Check sheet for the modelled part. Datum: model origin and axes. Units: mm. A direction names the side the tool comes from. Round coordinates to 2 decimals unless told otherwise and drop trailing zeros. Write each loop counter-clockwise with the first axis right and the second up, starting at its lowest first coordinate (ties: lowest second). Pieces come first, ordered by that corner, then holes. Notation, with made-up numbers: M -6.5,-17 L 10.5,-17 A12 cw 10.5,-9 Z; hole C 33.5,-19.5 d4. An arc over 180 degrees is marked long. Answer in a Markdown table with one row per item.
```python
from build123d import *

# Parameters (mm, degrees)
SKETCH1_W                = 34
SKETCH1_H                = 15
BOSS_EXTRUDE1_DEPTH      = 30
BOSS_EXTRUDE2_DEPTH      = 7
BOSS_EXTRUDE2_DEPTH_BACK = 37
CUT_EXTRUDE2_DEPTH       = 38
CUT_EXTRUDE3_DEPTH       = 6
CUT_EXTRUDE3_DEPTH_BACK  = 40
SKETCH7_R                = 2.75
CUT_EXTRUDE4_DEPTH       = 25.660254038


with BuildPart() as part:
    # Sketch1 → Boss-Extrude1 (new body)
    with BuildSketch(Plane.XY):
        with Locations((17, 7.5)):
            Rectangle(SKETCH1_W, SKETCH1_H)
    extrude(amount=BOSS_EXTRUDE1_DEPTH)

    # Sketch3 → Boss-Extrude2 (add, two sides)
    with BuildSketch(Plane.XY.offset(30)) as boss_extrude2_sk:
        Polygon((0, 0), (-5, -8.660254038), (-5, -9.660254038), (39, -9.660254038), (39, -8.660254038), (34, 0), align=None)
    extrude(amount=BOSS_EXTRUDE2_DEPTH)
    extrude(boss_extrude2_sk.sketch, amount=-BOSS_EXTRUDE2_DEPTH_BACK)

    # Sketch5 → Cut-Extrude2 (cut, through all)
    with BuildSketch(Plane.XY.offset(30)):
        Polygon((8, 4.324573519), (10.75, 5.91228676), (10.75, 9.08771324), (8, 10.675426481), (5.25, 9.08771324), (5.25, 5.91228676), align=None)
        Polygon((26, 4.324573519), (28.75, 5.91228676), (28.75, 9.08771324), (26, 10.675426481), (23.25, 9.08771324), (23.25, 5.91228676), align=None)
    extrude(amount=-CUT_EXTRUDE2_DEPTH, mode=Mode.SUBTRACT)

    # Sketch6 → Cut-Extrude3 (cut, two sides)
    with BuildSketch(Plane.ZY) as cut_extrude3_sk:
        Polygon((30, 0), (37, -8.660254038), (37, 0), align=None)
        Polygon((0, 0), (-7, -8.660254038), (-7, 0), align=None)
    extrude(amount=CUT_EXTRUDE3_DEPTH, mode=Mode.SUBTRACT)
    extrude(cut_extrude3_sk.sketch, amount=-CUT_EXTRUDE3_DEPTH_BACK, mode=Mode.SUBTRACT)

    # Sketch7 → Cut-Extrude4 (cut, through all)
    with BuildSketch(Plane(origin=(0, 15, 0), x_dir=(1, 0, 0), z_dir=(0, 1, 0))):
        with Locations((17, -6)):
            Circle(SKETCH7_R)
        with Locations((17, -24)):
            Circle(SKETCH7_R)
    extrude(amount=-CUT_EXTRUDE4_DEPTH, mode=Mode.SUBTRACT)


solid = part.part
```
1. Section check C-C, the plane z = 2. Record the cut outline in (x, y).
Found:
| item | result |
|---|---|
| outline | M -5,-9.66 L 39,-9.66 L 39,-8.66 L 34,0 L 34,15 L 0,15 L 0,0 L -5,-8.66 Z; hole M 5.25,5.91 L 8,4.32 L 10.75,5.91 L 10.75,9.09 L 8,10.68 L 5.25,9.09 Z; hole M 23.25,5.91 L 26,4.32 L 28.75,5.91 L 28.75,9.09 L 26,10.68 L 23.25,9.09 Z |
2. Section check B-B, the plane x = 17. Record the cut outline in (y, z), and give its area (3 significant figures).
Found:
| item | result |
|---|---|
| outline | M -9.66,-7 L -8.66,-7 L 0,0 L 15,0 L 15,3.25 L -9.66,3.25 Z; M -9.66,8.75 L 15,8.75 L 15,21.25 L -9.66,21.25 Z; M -9.66,26.75 L 15,26.75 L 15,30 L 0,30 L -8.66,37 L -9.66,37 Z |
| area | 543 mm2 |
3. Go/stop test with flat-tipped pins: pin 1 (1.6 mm diameter, centred on y = 8, z = 12, fed in from -X); pin 2 (1.5 mm diameter, centred on x = 16.5, y = -0.5, fed in from +Z); pin 3 (10 mm diameter, centred on x = 0, y = -7, fed in from -Z); pin 4 (10 mm diameter, centred on y = -2.5, z = 13.5, fed in from +X). Record where each tip stops, or that it passes through.
Found:
| item | result |
|---|---|
| pin 1 | stops at x = 0 |
| pin 2 | stops at z = 31.01 |
| pin 3 | stops at z = -7 |
| pin 4 | stops at x = 38.33 |
4. Scan lines: L1, parallel to Z at x = 17, y = 9.5; L2, parallel to X at y = 8.25, z = 24; L3, parallel to Z at x = 16, y = -2.75. Record each from-to range of solid material in increasing order.
Found:
| item | result |
|---|---|
| L1 | z = 0 to 3.25, 8.75 to 21.25, 26.75 to 30 |
| L2 | x = 0 to 5.25, 10.75 to 14.25, 19.75 to 23.25, 28.75 to 34 |
| L3 | z = -2.22 to 3.44, 8.56 to 21.44, 26.56 to 32.22 |
5. Access from +Z, -Z, +X, -X, +Y, -Y to the whole of each face (thin tool, end or side, straight path). Record for faces 4 (the face through (36.535, -4.391, 15.308)), 5 (the face through (0, 7, 15)), 6 (the face through (10.75, 7, 15)), 7 (the face through (17, 8, 30)).
Found:
| item | result |
|---|---|
| face 4 | +Z, -Z, +X, +Y |
| face 5 | +Z, -Z, -X, +Y |
| face 6 | +Z, -Z |
| face 7 | +Z, +X, -X, +Y |
6. Section check D-D, the plane y = 2.75. Record the cut outline in (x, z).
Found:
| item | result |
|---|---|
| outline | M 0,0 L 34,0 L 34,30 L 0,30 Z; hole C 17,6 d5.5; hole C 17,24 d5.5 |
7. Section check A-A, the plane z = 24. Record the cut outline in (x, y), and give its area (3 significant figures).
Found:
| item | result |
|---|---|
| outline | M -5,-9.66 L 14.25,-9.66 L 14.25,15 L 0,15 L 0,0 L -5,-8.66 Z; M 19.75,-9.66 L 39,-9.66 L 39,-8.66 L 34,0 L 34,15 L 19.75,15 Z; hole M 5.25,5.91 L 8,4.32 L 10.75,5.91 L 10.75,9.09 L 8,10.68 L 5.25,9.09 Z; hole M 23.25,5.91 L 26,4.32 L 28.75,5.91 L 28.75,9.09 L 26,10.68 L 23.25,9.09 Z |
| area | 704 mm2 |
8. Draft check along Z on faces 1 (the face through (17, -9.66, 15)), 2 (the face through (17, 8, 0)), 3 (the face through (16.642, 2.842, 21.273)). Enter one of: +Z half, -Z half, draft (parallel to the pull), parting line (faces both ways), or undercut.
Found:
| item | result |
|---|---|
| face 1 | draft |
| face 2 | -Z half |
| face 3 | undercut |
